Autodesk Inventor part; units mm, degrees
ref_plane "YZ Plane" through (0, 0, 0) normal (1, 0, 0) x (0, 1, 0)
ref_plane "XZ Plane" through (0, 0, 0) normal (0, 1, 0) x (-1, 0, 0)
ref_plane "XY Plane" through (0, 0, 0) normal (0, 0, 1) x (1, 0, 0)
sketch "Sketch1" plane through (0, 0, 0) normal (1, 0, 0) x (0, 1, 0)
  line L0 (12.5, 112.5) -> (12.5, -112.5)
  line L1 (12.5, -112.5) -> (-12.5, -112.5)
  line L2 (-12.5, -112.5) -> (-12.5, 112.5)
  line L3 (-12.5, 112.5) -> (12.5, 112.5)
  circle A0 centre (0, 100) radius 4
  circle A1 centre (0, -100) radius 4
  point P0 (0, 0)
  point P1 (-12.5, 94)
  point P2 (-12.5, 97.9432)
  dimension "d0" = 225
  dimension "d1" = 25
  dimension "d2" = 12.5
  dimension "d3" = 112.5
  dimension "d4" = 8
  dimension "d5" = 12.5
  dimension "d6" = 8
  dimension "d7" = 12.5
extrude "Extrusion1" add sketch "Sketch1" along normal blind 6
full round fillet "Full Round Fillet1" first side at (2, 12.5, -37.5) centre faces at (2, 4.1667, 112.5) second side at (2, -12.5, 37.5)
full round fillet "Full Round Fillet2" first side at (2, 12.5, -41.6666) centre faces at (2, -4.1667, -112.5) second side at (2, -12.5, 29.1667)
thread "Thread3"
thread "Thread4"
properties part number "Braço Macaco" material "Steel AISI 1050"
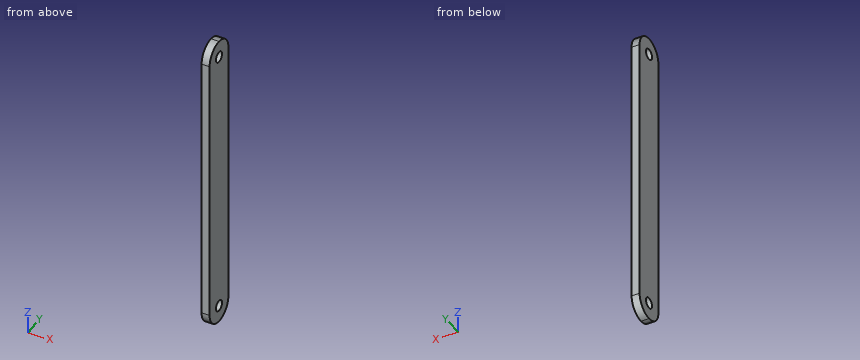
Build history of the part. All positions in model axes, mm. Give positions to 0.01 mm unless a question says otherwise; leave off trailing zeros. Loops run counter-clockwise (first coordinate to the right, second up) from the corner with the lowest first, then second, coordinate; pieces in that order, holes last.
1) Band-saw the part on A-A on x = 3.55. State how many separate pieces and enclosed holes the cut face has, then the cut area to 3 significant figures.
Values follow:
separate pieces: 1
enclosed holes: 2
area: 5,390 mm2
2) Band-saw the part on B-B on y = 7. List the corners of the cut face in (x, z).
Values follow:
outline: (0, -110.36) - (6, -110.36) - (6, 110.36) - (0, 110.36) - close
3) Drop flat-ended pins along their axis: P1, Ø3, axis at y = -8.5, z = -45.5, coming from the -X side; P2, Ø5, axis at y = 0, z = -100, coming from the -X side; P3, Ø2, axis at x = 5, y = 6.5, coming from the -Z side (3 decimals). Give the stop position or say it passes through.
Values follow:
P1: stops at x = 0
P2: passes through
P3: stops at z = -111.225
4) Probe line 1 along Z through (x, y) = (3.85, 0); line 2 along Z through (x, y) = (2.4, 1.25); line 3 along Z through (x, y) = (0.65, -10). List the from-to ranges inside material, lowest first.
Values follow:
line 1: z = -112.5 to -104, -96 to 96, 104 to 112.5
line 2: z = -112.44 to -103.8, -96.2 to 96.2, 103.8 to 112.44
line 3: z = -107.5 to 107.5
